from build123d import *

# Parameters (mm, degrees)
F0_R     = 4.2
F1_DEPTH = 20
F2_R     = 0.5
F3_DEPTH = 4.5
F4_R     = 0.5
F5_DEPTH = 30.6324


with BuildPart() as f1:
    # F0 (on Top) → F1 (new body)
    with BuildSketch(Plane.XY):
        Circle(F0_R)
    extrude(amount=F1_DEPTH)

    # F2 (on face) → F3 (join)
    with BuildSketch(Plane(origin=(0, 0, 0), x_dir=(1, 0, 0), z_dir=(0, 0, -1))):
        Circle(F2_R)
    extrude(amount=F3_DEPTH)

    # F4 (on face) → F5 (join)
    with BuildSketch(Plane(origin=(0, 0, -4.5), x_dir=(1, 0, 0), z_dir=(0, 0, -1))):
        Circle(F4_R)
    extrude(amount=-F5_DEPTH)


solid = f1.part
Part model, mm, in its own coordinate system. A direction names the side the tool comes from. Coordinates: 2 decimals unless noted, no trailing zeros. Loops run counter-clockwise (first coordinate to the right, second up) from the corner with the lowest first, then second, coordinate; pieces in that order, holes last. Notation, with made-up numbers: M -39,6.5 L 9,6.5 A19 ccw 9,15.5 Z; hole C 32.25,55 d2. An arc over 180 degrees is marked long. Use a Markdown table: item, result. Add a question column.
Q1. Probe L1, parallel to Z at x = -2.5, y = -2; L2, parallel to X at y = -0.25, z = 5.5; L3, parallel to Y at x = 3.75, z = 12. List the from-to ranges inside material, lowest first.
Q2. Cut at C-C (z = 14). Write the cut outline in (x, y).
Q3. Cut at D-D (z = 22). Write the cut outline in (x, y), and give its area (3 significant figures).
Q4. Which spindle directions (+Z, -Z, +X, -X, +Y, -Y) get a long thin tool onto all of the face, cutting with end or side? Do faces 1 (the cylindrical face through (-0.108, 0.488, 23.023)), 2 (the cylindrical face through (-0.108, 0.488, -2.218)), 3 (the flat face through (0, 0, -4.5)). Say none if no direction does.
Q5. Cut at A-A (y = 0). Write the cut outline in (x, z), and give its area (3 significant figures).
Q6. Pin check, flat tips, straight feed: P1, Ø5, axis at x = -3, z = 12, coming from the +Y side; P2, Ø5, axis at y = 3, z = 5.5, coming from the +X side. Stop position of each tip, or through.
Worked out:
| question | item | result |
|---|---|---|
| 1 | L1 | z = 0 to 20 |
| 1 | L2 | x = -4.19 to 4.19 |
| 1 | L3 | y = -1.89 to 1.89 |
| 2 | outline | C 0,0 d8.4 |
| 3 | outline | C 0,0 d1 |
| 3 | area | 0.785 mm2 |
| 4 | face 1 | +Z |
| 4 | face 2 | -Z |
| 4 | face 3 | -Z, +X, -X, +Y, -Y |
| 5 | outline | M -4.2,0 L -0.5,0 L -0.5,-4.5 L 0.5,-4.5 L 0.5,0 L 4.2,0 L 4.2,20 L 0.5,20 L 0.5,26.13 L -0.5,26.13 L -0.5,20 L -4.2,20 Z |
| 5 | area | 179 mm2 |
| 6 | P1 | stops at y = 4.17 |
| 6 | P2 | stops at x = 4.17 |
